```python
from build123d import *

# Parameters (mm, degrees)
SKIZZE1_W                       = 90
SKIZZE1_H                       = 60
AUFSATZ_LINEAR_AUSTRAGEN1_DEPTH = 5
SKIZZE2_W                       = 90
SKIZZE2_H                       = 5
AUFSATZ_LINEAR_AUSTRAGEN2_DEPTH = 40
SKIZZE3_W                       = 45
SKIZZE3_H                       = 4
AUFSATZ_LINEAR_AUSTRAGEN3_DEPTH = 37
SKIZZE4_R                       = 2.1
SKIZZE4_W                       = 20
SKIZZE4_H                       = 10
SCHNITT_LINEAR_AUSTRAGEN1_DEPTH = 5
FASE1_SIZE                      = 2
FASE2_SIZE                      = 2
SKIZZE6_R                       = 3.5
SCHNITT_LINEAR_AUSTRAGEN2_DEPTH = 5
SCHNITT_LINEAR_START            = -5
SKIZZE8_R                       = 3.5
SCHNITT_LINEAR_AUSTRAGEN3_DEPTH = 5
SKIZZE9_R                       = 1.65
SCHNITT_LINEAR_AUSTRAGEN4_DEPTH = 5
FASE3_SIZE                      = 2
SKIZZE10_W                      = 30
SKIZZE10_H                      = 40
SCHNITT_LINEAR_AUSTRAGEN5_DEPTH = 10
SKIZZE11_W                      = 12.5
SKIZZE11_H                      = 5.996169329
SCHNITT_LINEAR_AUSTRAGEN6_DEPTH = 10
SKIZZE12_W                      = 10
SKIZZE12_H                      = 40
SCHNITT_LINEAR_AUSTRAGEN7_DEPTH = 10


with BuildPart() as part:
    # Skizze1 → Aufsatz-Linear austragen1 (new body)
    with BuildSketch(Plane(origin=(0, 0, 0), x_dir=(1, 0, 0), z_dir=(0, 1, 0))):
        Rectangle(SKIZZE1_W, SKIZZE1_H)
    extrude(amount=AUFSATZ_LINEAR_AUSTRAGEN1_DEPTH)

    # Skizze2 → Aufsatz-Linear austragen2 (add)
    with BuildSketch(Plane(origin=(0, 5, 0), x_dir=(1, 0, 0), z_dir=(0, 1, 0))):
        with Locations((0, 27.5)):
            Rectangle(SKIZZE2_W, SKIZZE2_H)
        with Locations((0, -27.5)):
            Rectangle(SKIZZE2_W, SKIZZE2_H)
    extrude(amount=AUFSATZ_LINEAR_AUSTRAGEN2_DEPTH)

    # Skizze3 → Aufsatz-Linear austragen3 (add)
    with BuildSketch(Plane(origin=(0, 5, 0), x_dir=(1, 0, 0), z_dir=(0, 1, 0))):
        with Locations((-22.5, 11.004200432)):
            Rectangle(SKIZZE3_W, SKIZZE3_H)
    extrude(amount=AUFSATZ_LINEAR_AUSTRAGEN3_DEPTH)

    # Skizze4 → Schnitt-Linear austragen1 (cut)
    with BuildSketch(Plane.XY.offset(-9.004200432)):
        with Locations((-40, 32)):
            Circle(SKIZZE4_R)
        with Locations((-5, 32)):
            Circle(SKIZZE4_R)
        with Locations((-22.5, 37)):
            Rectangle(SKIZZE4_W, SKIZZE4_H)
    extrude(amount=-SCHNITT_LINEAR_AUSTRAGEN1_DEPTH, mode=Mode.SUBTRACT)

    # Fase1
    fase1_edges = [part.edges().sort_by_distance(p)[0] for p in [
        (-42.1, 32, -13.004200432),
    ]]
    chamfer(fase1_edges, length=FASE1_SIZE)

    # Fase2
    fase2_edges = [part.edges().sort_by_distance(p)[0] for p in [
        (-7.1, 32, -13.004200432),
    ]]
    chamfer(fase2_edges, length=FASE2_SIZE)

    # Skizze6 → Schnitt-Linear austragen2 (cut)
    with BuildSketch(Plane(origin=(0, 0, -30), x_dir=(-1, 0, 0), z_dir=(0, 0, -1))):
        with Locations((-15, 40)):
            Circle(SKIZZE6_R)
    extrude(amount=-SCHNITT_LINEAR_AUSTRAGEN2_DEPTH, mode=Mode.SUBTRACT)

    # Skizze8 → Schnitt-Linear austragen3 (cut)
    with BuildSketch(Plane.XY.offset(30).offset(SCHNITT_LINEAR_START)):
        with Locations(Location((15, 40, 0), (0, 0, 180))):
            Circle(SKIZZE8_R)
    extrude(amount=SCHNITT_LINEAR_AUSTRAGEN3_DEPTH, mode=Mode.SUBTRACT)

    # Skizze9 → Schnitt-Linear austragen4 (cut)
    with BuildSketch(Plane(origin=(0, 5, 0), x_dir=(1, 0, 0), z_dir=(0, 1, 0))):
        with Locations(Location((35, 5, 0), (0, 0, 270))):
            Circle(SKIZZE9_R)
        with Locations(Location((35, -15, 0), (0, 0, 270))):
            Circle(SKIZZE9_R)
        with Locations(Location((-35, -15, 0), (0, 0, 270))):
            Circle(SKIZZE9_R)
        with Locations(Location((-35, 5, 0), (0, 0, 270))):
            Circle(SKIZZE9_R)
    extrude(amount=-SCHNITT_LINEAR_AUSTRAGEN4_DEPTH, mode=Mode.SUBTRACT)

    # Fase3
    fase3_edges = [part.edges().sort_by_distance(p)[0] for p in [
        (-35, 5, -6.65),
        (-35, 5, 13.35),
        (35, 5, 13.35),
        (35, 5, -6.65),
    ]]
    chamfer(fase3_edges, length=FASE3_SIZE)

    # Skizze10 → Schnitt-Linear austragen5 (cut)
    with BuildSketch(Plane.XY.offset(30)):
        with Locations((-30, 25)):
            Rectangle(SKIZZE10_W, SKIZZE10_H)
    extrude(amount=-SCHNITT_LINEAR_AUSTRAGEN5_DEPTH, mode=Mode.SUBTRACT)

    # Skizze11 → Schnitt-Linear austragen6 (cut)
    with BuildSketch(Plane.XY.offset(-9.004200432)):
        with Locations((-38.75, 39.001915336)):
            Rectangle(SKIZZE11_W, SKIZZE11_H)
    extrude(amount=-SCHNITT_LINEAR_AUSTRAGEN6_DEPTH, mode=Mode.SUBTRACT)

    # Skizze12 → Schnitt-Linear austragen7 (cut)
    with BuildSketch(Plane(origin=(0, 0, -30), x_dir=(-1, 0, 0), z_dir=(0, 0, -1))):
        with Locations((40, 25)):
            Rectangle(SKIZZE12_W, SKIZZE12_H)
    extrude(amount=-SCHNITT_LINEAR_AUSTRAGEN7_DEPTH, mode=Mode.SUBTRACT)


solid = part.part
```
Verification items for the finished model (mm, model axes). A direction names the side the tool comes from. Give positions to 0.01 mm unless a question says otherwise; leave off trailing zeros. Order: outer loops, then holes, each group sorted by start corner. A loop starts at its lowest first (then second) coordinate and runs counter-clockwise, first axis right, second up. Notation, with made-up numbers: (73, -2) -> (114, -2) arc R10 cw to (114, 11) -> close; hole circle Ø4 at (44.5, 2.25). An arc over 180 degrees is marked (long way). One line per item, written item: value.
(1) Sectioned sample at A-A on x = 35. Record the cut outline in (y, z), then the cut area to 3 significant figures.
Final values:
outline: (0, -30) -> (45, -30) -> (45, -25) -> (5, -25) -> (5, -8.65) -> (3, -6.65) -> (0, -6.65) -> close; (0, -3.35) -> (3, -3.35) -> (5, -1.35) -> (5, 11.35) -> (3, 13.35) -> (0, 13.35) -> close; (0, 16.65) -> (3, 16.65) -> (5, 18.65) -> (5, 25) -> (45, 25) -> (45, 30) -> (0, 30) -> close
area: 659 mm^2
(2) Sectioned sample at B-B on y = 40. Record the cut outline in (x, z), then the cut area to 3 significant figures.
Final values:
outline: (-35, -30) -> (11.5, -30) -> (11.5, -25) -> (-35, -25) -> close; (-15, 25) -> (11.5, 25) -> (11.5, 30) -> (-15, 30) -> close; (-12.5, -13) -> (0, -13) -> (0, -9) -> (-12.5, -9) -> close; (18.5, -30) -> (45, -30) -> (45, -25) -> (18.5, -25) -> close; (18.5, 25) -> (45, 25) -> (45, 30) -> (18.5, 30) -> close
area: 680 mm^2
(3) Sectioned sample at D-D on y = 24.5. Record the cut outline in (x, z).
Final values:
outline: (-45, -13) -> (0, -13) -> (0, -9) -> (-45, -9) -> close; (-35, -30) -> (45, -30) -> (45, -25) -> (-35, -25) -> close; (-15, 25) -> (45, 25) -> (45, 30) -> (-15, 30) -> close
(4) Draft check along Y on faces 1 (the face through (-23, 32, -11)), 2 (the face through (15, 25, 25)), 3 (the face through (-40.46, 29.95, -9.99)), 4 (the face through (-1, 0, 0)). Enter one of: pulls with the +Y half, pulls with the -Y half, needs draft (parallel to the pull), parting line crosses it, or undercut.
Final values:
face 1: pulls with the +Y half
face 2: needs draft
face 3: undercut
face 4: pulls with the -Y half
(5) Scan lines: line 1 along Z through (x, y) = (-9, 9); line 2 along X through (y, z) = (1.2, -5); line 3 along Y through (x, z) = (15, -28.55). Record each from-to range of solid material in increasing order. Write a range as [from, to].
Final values:
line 1: [-30, -25], [-13, -9], [25, 30]
line 2: [-45, -36.65], [-33.35, 33.35], [36.65, 45]
line 3: [0, 36.5], [43.5, 45]
(6) Sectioned sample at C-C on z = 15. Record the cut outline in (x, y), then the cut area to 3 significant figures.
Final values:
outline: (-45, 0) -> (-36.65, 0) -> (-36.65, 3) -> (-38.65, 5) -> (-45, 5) -> close; (-33.35, 0) -> (33.35, 0) -> (33.35, 3) -> (31.35, 5) -> (-31.35, 5) -> (-33.35, 3) -> close; (36.65, 0) -> (45, 0) -> (45, 5) -> (38.65, 5) -> (36.65, 3) -> close
area: 409 mm^2
(7) Gauge pin test, flat ends, axial feed: pin 1 (2 mm diameter, centred on y = 34.5, z = -11, fed in from +X); pin 2 (2 mm diameter, centred on x = -25.5, y = 38.5, fed in from +Z); pin 3 (5.5 mm diameter, centred on y = 28, z = 27.5, fed in from -X); pin 4 (12 mm diameter, centred on y = 33.5, z = -19.5, fed in from +X). Record the tip position at first contact, or that the pin passes through.
Final values:
pin 1: x = 0
pin 2: z = -25
pin 3: x = -15
pin 4: x = 45
(8) Tool access check on faces 5 (the face through (-35, 25, -28)), 6 (the face through (-12.5, 37, -11)), 7 (the face through (-5.46, 29.95, -9.99)), 8 (the face through (-15, 25, 28)), 9 (the face through (-32.5, 34, -11)). Record the directions out of +Z, -Z, +X, -X, +Y, -Y that give a thin tool (end or side, any length) a straight path to the whole face; none if there is none.
Final values:
face 5: -Z, -X, +Y
face 6: +Y
face 7: none
face 8: +Z, -X, +Y
face 9: +Z, +Y
